from build123d import *

# Parameters (mm, degrees)
F1_R          = 8
F1_R_2        = 2.35
F2_DEPTH      = 1
F3_DEPTH      = 7
F4_DEPTH      = 1.1
F4_DEPTH_BACK = 0.1016
F7_R          = 3.280158
F7_R_2        = 2.35
F8_DEPTH      = 1


with BuildPart() as f2:
    # F1 (on Top) → F2 (new body)
    with BuildSketch(Plane.XY):
        with Locations((0, 28.162442)):
            Circle(F1_R)
        with Locations((0, 28.162442)):
            Circle(F1_R_2, mode=Mode.SUBTRACT)
        with Locations((0, 28.162442)):
            Circle(F1_R_2)
    extrude(amount=F2_DEPTH)

    # F1 (on Top) → F3 (join)
    with BuildSketch(Plane.XY):
        with Locations((0, 28.162442)):
            Circle(F1_R_2)
    extrude(amount=F3_DEPTH)

    # F7 (on face) → F8 (join)
    with BuildSketch(Plane.XY.offset(1)):
        with Locations((0, 28.162442)):
            Circle(F7_R)
        with Locations((0, 28.162442)):
            Circle(F7_R_2, mode=Mode.SUBTRACT)
    extrude(amount=F8_DEPTH)


with BuildPart() as f4:
    # F1 (on Top) → F4 (new body, two sides)
    with BuildSketch(Plane.XY) as f4_sk:
        with Locations((0, 28.162442)):
            Circle(F1_R)
        with Locations((0, 28.162442)):
            Circle(F1_R_2, mode=Mode.SUBTRACT)
        with Locations((0, 28.162442)):
            Circle(F1_R_2)
    extrude(amount=-F4_DEPTH)
    extrude(f4_sk.sketch, amount=-F4_DEPTH_BACK)


with BuildPart() as f4_1:
    # F5: moved
    add(f4.part.moved(Location((-18.7706, 0, 1.0922))))


solid = f2.part
CAD build for the part. Positions are in the model's coordinates, mm. A direction names the side the tool comes from. Give positions to 0.01 mm unless a question says otherwise; leave off trailing zeros. Write each loop counter-clockwise with the first axis right and the second up, starting at its lowest first coordinate (ties: lowest second). Pieces come first, ordered by that corner, then holes. Notation, with made-up numbers: M 82.5,61.25 L 120.5,61.25 A25 ccw 120.5,88.25 Z; hole C -22,47.5 d9. An arc over 180 degrees is marked long. Put each result on its own line as item: value. Start each with the question number.
(1) Probe L1, parallel to Z at x = 1.75, y = 30.5; L2, parallel to Z at x = -1, y = 21.25; L3, parallel to X at y = 30.25, z = 4.25. List the from-to ranges inside material, lowest first.
(2) Band-saw the part on A-A, the plane x = 0. Write the cut outline in (y, z).
(3) Band-saw the part on B-B, the plane y = 27.5. Write the cut outline in (x, z).
(4) Band-saw the part on D-D, the plane z = 4. Write the cut outline in (x, y).
(5) Flat gauge pin, fed straight in: pin 1 Ø1.5 at (y, z) = (32, 1) entering from -X. Where does the tip first touch, or does it go through?
(6) Band-saw the part on C-C, the plane y = 30.75. Write the cut outline in (x, z), and give its area (3 significant figures).
(7) Which spindle directions (+Z, -Z, +X, -X, +Y, -Y) get a long thin tool onto all of the face, cutting with end or side? Do faces 1 (the face through (0, 28, 0)), 2 (the face through (-0.427, 31.415, 1.493)). Say none if no direction does.
Response values:
1. L1: z = 0 to 2
1. L2: z = 0 to 1
1. L3: x = -1.08 to 1.08
2. outline: M 20.16,0 L 36.16,0 L 36.16,1 L 31.44,1 L 31.44,2 L 30.51,2 L 30.51,7 L 25.81,7 L 25.81,2 L 24.88,2 L 24.88,1 L 20.16,1 Z
3. outline: M -7.97,0 L 7.97,0 L 7.97,1 L 3.21,1 L 3.21,2 L 2.25,2 L 2.25,7 L -2.25,7 L -2.25,2 L -3.21,2 L -3.21,1 L -7.97,1 Z
4. outline: C 0,28.16 d4.7
5. pin 1: stops at x = -7.38
6. outline: M -7.57,0 L 7.57,0 L 7.57,1 L 2.02,1 L 2.02,2 L -2.02,2 L -2.02,1 L -7.57,1 Z
6. area: 19.2 mm2
7. face 1: -Z, +X, -X, +Y, -Y
7. face 2: +Z
